from build123d import *

# Parameters (mm, degrees)
F0_W     = 63
F0_H     = 21.5
F1_DEPTH = 5
F3_DEPTH = 58
F4_DEPTH = 63.001
F6_DEPTH = 20


with BuildPart() as f1:
    # F0 (on Right) → F1 (new body)
    with BuildSketch(Plane.YZ):
        Rectangle(F0_W, F0_H)
    extrude(amount=F1_DEPTH)

    # F2 (on face) → F3 (cut)
    with BuildSketch(Plane.XZ.offset(31.5)):
        with BuildLine():
            Line((5, 7.25), (5, 9.25))
            ThreePointArc((5, 9.25), (4, 8.25), (5, 7.25))
        make_face()
    extrude(amount=-F3_DEPTH, mode=Mode.SUBTRACT)

    # F2 (on face) → F4 (cut, through all)
    with BuildSketch(Plane.XZ.offset(31.5)):
        Polygon((1.5, -9.25), (0, -9.25), (0, -10.75), (1, -10.75), align=None)
        Polygon((3.5, -9.25), (4, -10.75), (5, -10.75), (5, -9.25), align=None)
    extrude(amount=-F4_DEPTH, mode=Mode.SUBTRACT)

    # F5 (on face) → F6 (cut, through all)
    with BuildSketch(Plane.XY.offset(10.75)):
        Polygon((5, 28.5), (5, 30), (3.5, 30.5), (3.5, 28), align=None)
    extrude(amount=-F6_DEPTH, mode=Mode.SUBTRACT)


solid = f1.part
Can you work these out from the model? Positions are in its coordinate system, mm. A direction names the side the tool comes from. Give positions to 0.01 mm unless a question says otherwise; leave off trailing zeros. Write each loop counter-clockwise with the first axis right and the second up, starting at its lowest first coordinate (ties: lowest second). Pieces come first, ordered by that corner, then holes. Notation, with made-up numbers: M -2.75,49.25 L 46.25,49.25 A13 ccw 46.25,63.25 Z; hole C 27,-3 d4. An arc over 180 degrees is marked long. Answer in a Markdown table with one row per item. Add a question column.
Item 1: Please list where these lines run through material, in increasing order: L1, parallel to Y at x = 3.85, z = -8; L2, parallel to Y at x = 4.45, z = 4; L3, parallel to Z at x = 4.2, y = 10.
Item 2: Imagine slicing it at B-B, the plane z = 8.25. Write out the boundary of the cut face in (x, y).
Item 3: Imagine slicing it at A-A, the plane y = -5.5. Write out the boundary of the cut face in (x, z), plus the area to 3 significant figures.
Item 4: We'd pull the mould along X, two halves only. Please class faces 1 (the flat face through (2, 0, 10.75)), 2 (the flat face through (3.5, 29, 1)), 3 (the flat face through (1.247, -0.441, -10.01)): released by +X, released by -X, zero draft, split by the parting line, or undercut.
Item 5: On a 3-axis mill with a long thin cutter (end or side, diameter ignored), from which of +Z, -Z, +X, -X, +Y, -Y can I reach the whole of each face in a straight line? I mean faces 4 (the cylindrical face through (4, -2.9, 8.3)), 5 (the flat face through (5, 31, 1)), 6 (the flat face through (4.24, 28.246, 0.89)), 7 (the flat face through (4, 31, -9.25)), 8 (the flat face through (2, 31.5, 0)). Say none if no direction works.
Evaluation:
| question | item | result |
|---|---|---|
| 1 | L1 | y = -31.5 to 28.12, 30.38 to 31.5 |
| 1 | L2 | y = -31.5 to 28.32, 30.18 to 31.5 |
| 1 | L3 | z = -9.25 to 7.65, 8.85 to 10.75 |
| 2 | outline | M 0,-31.5 L 4,-31.5 L 4,26.5 L 5,26.5 L 5,28.5 L 3.5,28 L 3.5,30.5 L 5,30 L 5,31.5 L 0,31.5 Z |
| 3 | outline | M 0,-9.25 L 1.5,-9.25 L 1,-10.75 L 4,-10.75 L 3.5,-9.25 L 5,-9.25 L 5,7.25 A1 cw 5,9.25 L 5,10.75 L 0,10.75 Z |
| 3 | area | 102 mm² |
| 4 | face 1 | zero draft |
| 4 | face 2 | undercut |
| 4 | face 3 | released by -X |
| 5 | face 4 | +X, -Y |
| 5 | face 5 | +Z, -Z, +X, +Y, -Y |
| 5 | face 6 | +Z |
| 5 | face 7 | +X, +Y, -Y |
| 5 | face 8 | +Z, -Z, +X, -X, +Y |
